The model under review builds one solid part; all positions refer to its coordinate system, in mm. Face numbers are marked on the shaded views. A direction names the side the tool comes from. Coordinates: 2 decimals unless noted, no trailing zeros. Loops run counter-clockwise (first coordinate to the right, second up) from the corner with the lowest first, then second, coordinate; pieces in that order, holes last. Notation, with made-up numbers: (-38.75, -28.5) - (-2.75, -28.5) arc R20 cw to (-2.75, -17.5) - close; hole circle Ø5 at (12.25, 7). An arc over 180 degrees is marked (long way). Answer in a Markdown table with one row per item. Add a question column.
(1) We need section B-B on y = 10.5. Write out the cut boundary in (x, z).
(2) We need section A-A on y = 17. Write out the cut boundary in (x, z), plus the area to 3 significant figures.
(3) Machinability: for the marked faces 1, 2, 3 and 4, which of the approach directions +Z, -Z, +X, -X, +Y, -Y give a long, thin tool a straight path to every point of the face, cutting with its end or side? Answer none if there is none.
(4) For P1, Ø0.6, axis at y = 1, z = -2, coming from the +X side; P2, Ø6, axis at x = 3.5, y = 16.5, coming from the -Z side; P3, Ø4, axis at x = -0.5, z = -1, coming from the +Y side; P4, Ø4, axis at y = 14, z = 1, coming from the +X side, all flat-tipped, find the tip position at first contact; note any pin that passes through.
(5) Mouldability with a two-part tool opening along Y and no side actions: class the marked faces 5, 6 and 7 as +Y half, -Y half, draft (parallel to the pull), parting line (faces both ways), or undercut.
(6) For line 1 along Z through (x, y) = (0, 0.2); line 2 along Y through (x, z) = (-3.25, 6); line 3 along X through (y, z) = (0.2, 0), list the stretches that pass through material, from the lowest coordinate up.
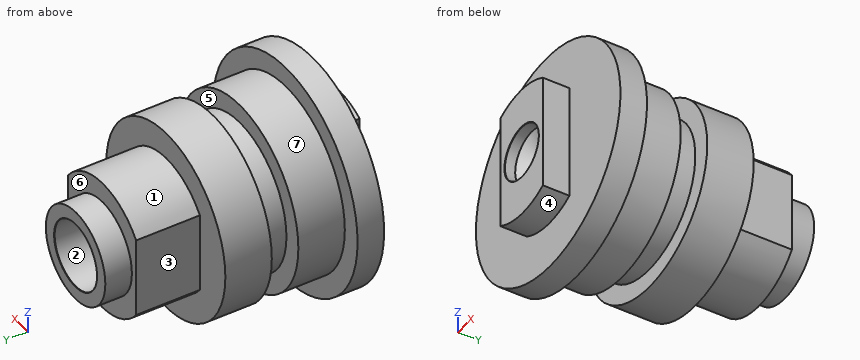
from build123d import *

# Parameters (mm, degrees)
CUT_EXTRUDE_1_DEPTH = 4.8
CUT_EXTRUDE_START   = -2
CUT_EXTRUDE_2_DEPTH = 2
MM_1_D              = 5
MM_1_DEPTH          = 5.497848452
MM_1_CSINK_D        = 5.05
MM_1_CSINK_ANGLE    = 90
MM_1_TIP            = 1.502151548


with BuildPart() as part:
    # 草图1 → 旋转1 (revolve)
    with BuildSketch(Plane.XY, mode=Mode.PRIVATE) as revolve_1_sk:
        Polygon((0, 0), (5, 0), (5, 2), (8.5, 2), (8.5, 4), (7, 4), (7, 7.5), (5.6, 7.5), (5.6, 9.5), (7, 9.5), (7, 13), (5, 13), (5, 17.8), (3.5, 17.8), (3.5, 19.8), (0, 19.8), align=None)
    revolve(revolve_1_sk.sketch.rotate(Axis((0, 19.8, 0), (0, -1, 0)), 180), axis=Axis((0, 19.8, 0), (0, -1, 0)))

    # 草图3 → 切除-拉伸1 (cut)
    with BuildSketch(Plane(origin=(0, 17.8, 0), x_dir=(1, 0, 0), z_dir=(0, 1, 0))):
        with BuildLine():
            Line((-4, 3), (-4, -3))
            ThreePointArc((-4, -3), (-5, 0), (-4, 3))
        make_face()
        with BuildLine():
            Line((4, 3), (4, -3))
            ThreePointArc((4, -3), (5, 0), (4, 3))
        make_face()
    extrude(amount=-CUT_EXTRUDE_1_DEPTH, mode=Mode.SUBTRACT)

    # 草图4 → 切除-拉伸2 (cut)
    with BuildSketch(Plane.XZ.offset(CUT_EXTRUDE_START)):
        with BuildLine():
            Line((-2.5, 4.330127019), (-2.5, -4.330127019))
            ThreePointArc((-2.5, -4.330127019), (-5, 0), (-2.5, 4.330127019))
        make_face()
        with BuildLine():
            Line((2.5, 4.330127019), (2.5, -4.330127019))
            ThreePointArc((2.5, -4.330127019), (5, 0), (2.5, 4.330127019))
        make_face()
    extrude(amount=CUT_EXTRUDE_2_DEPTH, mode=Mode.SUBTRACT)

    # 草图6 → 大小mm 暗销孔2 (revolve, cut)
    with BuildSketch(Plane(origin=(0, 0, 0), x_dir=(0, 0, -1), z_dir=(1, 0, 0))):
        Polygon((0, 0), (0, 2), (2, 0.798278762), (2, 0.025), (2.025, 0), align=None)
    revolve(axis=Axis((0, -6.35, 0), (0, 1, 0)), mode=Mode.SUBTRACT)

    # 大小mm 暗销孔1
    with Locations(Plane(origin=(0, 19.8, 0), x_dir=(1, 0, 0), z_dir=(0, 1, 0))):
        with Locations((0, 0)):
            CounterSinkHole(MM_1_D / 2, MM_1_CSINK_D / 2, depth=MM_1_DEPTH, counter_sink_angle=MM_1_CSINK_ANGLE)
            with Locations((0, 0, -(MM_1_DEPTH + MM_1_TIP / 2))):  # 118° drill point
                Cone(0, MM_1_D / 2, MM_1_TIP, mode=Mode.SUBTRACT)


solid = part.part
Outcome:
| question | item | result |
|---|---|---|
| 1 | outline | circle Ø14 at (0, 0) |
| 2 | outline | (-4, -3) arc R5 ccw to (4, -3) - (4, 3) arc R5 ccw to (-4, 3) - close; hole circle Ø5 at (0, 0) |
| 2 | area | 50.7 mm² |
| 3 | face 1 | +Z, +Y |
| 3 | face 2 | +Y |
| 3 | face 3 | +Z, -Z, -X, +Y |
| 3 | face 4 | -Z, -Y |
| 4 | P1 | x = 2.5 |
| 4 | P2 | z = -4.97 |
| 4 | P3 | y = 19.8 |
| 4 | P4 | x = 7 |
| 5 | face 5 | undercut |
| 5 | face 6 | +Y half |
| 5 | face 7 | draft |
| 6 | line 1 | -5 to -2, 2 to 5 |
| 6 | line 2 | 2 to 7.5, 9.5 to 13 |
| 6 | line 3 | -2.5 to -2, 2 to 2.5 |
